Design review of the part built by this model. Coordinates are the model's own, in mm. A direction names the side the tool comes from. Coordinates: 2 decimals unless noted, no trailing zeros. Order: outer loops, then holes, each group sorted by start corner. A loop starts at its lowest first (then second) coordinate and runs counter-clockwise, first axis right, second up. Notation, with made-up numbers: (20.25, -20.75) -> (36.25, -20.75) arc R16 ccw to (36.25, -3.75) -> close; hole circle Ø3 at (9, 18.25). An arc over 180 degrees is marked (long way). Use a Markdown table: item, result. Add a question column.
Q1. Add section B-B (x = 51). State the section outline as (y, z) points.
Q2. Machinability: for faces 5 (the face through (42.22, 1.81, 1.88)), 6 (the face through (3.81, 20, -45)), 7 (the face through (66.802, 17, -44)), 8 (the face through (24.274, 1.865, 1.878)), 9 (the face through (33, 3.679, 2)), which of the approach directions +Z, -Z, +X, -X, +Y, -Y give a long, thin tool a straight path to every point of the face, cutting with its end or side? Answer none if there is none.
Q3. Add section C-C (z = -33). State the section outline as (x, y) points.
Q4. Add section A-A (y = 8.5). State the section outline as (x, z) points, then the cut area to 3 significant figures.
Q5. Wall thickness on probe 1 along X at (y, z) = (25.5, -57.5); probe 2 along Z at (x, y) = (19.5, 23); probe 3 along Y at (x, z) = (4.5, -35.5): over which ranges is each line inside the solid? List them lowest first.
Q6. Insertion check: pin 1 (1.5 mm diameter, centred on x = 8, z = -22, fed in from +Y); pin 2 (4 mm diameter, centred on x = 35.5, z = 2.5, fed in from +Y); pin 3 (3 mm diameter, centred on x = 50, y = 18, fed in from +Z). Each pin has a flat end and moves straight along its axis. Give the tip position at first contact, or say it passes through.
Q7. Add section D-D (x = 42). State the section outline as (y, z) points, then the cut area to 3 significant figures.
Q8. The part is to be moulded in two halves that separate along Z. For faces 1 (the face through (33, 18, -90.17)), 2 (the face through (33, 4.572, -46)), 3 (the face through (33, 18, 0)), 4 (the face through (3.6, 35.052, -44.9)), say which applies: pulls with the +Z half, pulls with the -Z half, needs draft (parallel to the pull), parting line crosses it, or undercut.
from build123d import *

# Parameters (mm, degrees)
SKETCH1_W           = 66.802
SKETCH1_H           = 35.052
BOSS_EXTRUDE1_DEPTH = 90.17
SKETCH2_W           = 59.182
SKETCH2_H           = 82.55
CUT_EXTRUDE2_DEPTH  = 30.48
BOSS_EXTRUDE2_DEPTH = 3.81


with BuildPart() as part:
    # Sketch1 → Boss-Extrude1 (new body)
    with BuildSketch(Plane.XY):
        with Locations((33.401, 17.526)):
            Rectangle(SKETCH1_W, SKETCH1_H)
    extrude(amount=-BOSS_EXTRUDE1_DEPTH)

    # Sketch2 → Cut-Extrude2 (cut)
    with BuildSketch(Plane(origin=(0, 35.052, 0), x_dir=(1, 0, 0), z_dir=(0, 1, 0))):
        with Locations((33.401, 45.085)):
            Rectangle(SKETCH2_W, SKETCH2_H)
    extrude(amount=-CUT_EXTRUDE2_DEPTH, mode=Mode.SUBTRACT)

    # Sketch3 → Boss-Extrude2 (add)
    with BuildSketch(Plane.XY):
        Polygon((26.781803903, 3.679405909), (21.695474271, 0), (33.226810629, 0), (44.758146987, 0), (39.602141606, 3.679405909), align=None)
    extrude(amount=BOSS_EXTRUDE2_DEPTH)


solid = part.part
Established:
| question | item | result |
|---|---|---|
| 1 | outline | (0, -90.17) -> (35.05, -90.17) -> (35.05, -86.36) -> (4.57, -86.36) -> (4.57, -3.81) -> (35.05, -3.81) -> (35.05, 0) -> (0, 0) -> close |
| 2 | face 5 | +Z, +X, +Y |
| 2 | face 6 | +Y |
| 2 | face 7 | +Z, -Z, +X, +Y, -Y |
| 2 | face 8 | +Z, -X, +Y |
| 2 | face 9 | +Z, +X, -X, +Y |
| 3 | outline | (0, 0) -> (66.8, 0) -> (66.8, 35.05) -> (62.99, 35.05) -> (62.99, 4.57) -> (3.81, 4.57) -> (3.81, 35.05) -> (0, 35.05) -> close |
| 4 | outline | (0, -90.17) -> (66.8, -90.17) -> (66.8, 0) -> (0, 0) -> close; hole (3.81, -86.36) -> (62.99, -86.36) -> (62.99, -3.81) -> (3.81, -3.81) -> close |
| 4 | area | 1,140 mm^2 |
| 5 | probe 1 | 0 to 3.81, 62.99 to 66.8 |
| 5 | probe 2 | -90.17 to -86.36, -3.81 to 0 |
| 5 | probe 3 | 0 to 4.57 |
| 6 | pin 1 | y = 4.57 |
| 6 | pin 2 | y = 3.68 |
| 6 | pin 3 | z = 0 |
| 7 | outline | (0, -90.17) -> (35.05, -90.17) -> (35.05, -86.36) -> (4.57, -86.36) -> (4.57, -3.81) -> (35.05, -3.81) -> (35.05, 0) -> (1.97, 0) -> (1.97, 3.81) -> (0, 3.81) -> close |
| 7 | area | 652 mm^2 |
| 8 | face 1 | pulls with the -Z half |
| 8 | face 2 | undercut |
| 8 | face 3 | pulls with the +Z half |
| 8 | face 4 | needs draft |
